Could you check a few things on this model? Use its own coordinates, in mm. Coordinates: 2 decimals unless noted, no trailing zeros. Loops run counter-clockwise (first coordinate to the right, second up) from the corner with the lowest first, then second, coordinate; pieces in that order, holes last. Notation, with made-up numbers: (48.25, 57.5) - (60.25, 57.5) arc R14 ccw to (60.25, 77.5) - close; hole circle Ø8 at (70.25, 32.5). An arc over 180 degrees is marked (long way). One line per item, written item: value. Start each with the question number.
(1) If we section it at A-A on z = 1.6: Count the separate pieces of the cut face and the enclosed holes in it, then the cut area to 3 significant figures.
(2) I'm going to push a flat-ended pin straight in: P1, Ø5.5, axis at x = 320.675, y = 0, coming from the +Z side. Where does the tip first touch, or does it pass through?
(3) If we mould it in two halves opening along X, with no side actions, what happens to faces 1 (the face through (58.89, 6.35, 1.57)), 2 (the face through (308.071, -14.845, 1.565)), 3 (the face through (119, -24, 3.175)), 4 (the face through (-81.46, -97.464, 1.565))? For each: pulls with the +X half, pulls with the -X half, needs draft (parallel to the pull), parting line crosses it, or undercut.
(4) If we section it at B-B on x = 210: Write out the boundary of the cut face in (y, z) (3 decimals).
(5) If I drill on line 1 along Y through (x, z) = (302.5, 2.7); line 2 along X through (y, z) = (0.5, 2.65); line 3 along X through (y, z) = (11, 1.15), over which ranges is the centre line in solid material (lowest first)? Write a range as from..to.
(6) If we section it at C-C on x = -39: Write out the boundary of the cut face in (y, z) (3 decimals).
```python
from build123d import *

# Parameters (mm, degrees)
SKETCH1_R           = 7.9375
SKETCH1_R_2         = 3.429
SKETCH1_R_3         = 14.2875
SKETCH1_R_4         = 3.556
BOSS_EXTRUDE1_DEPTH = 3.175


with BuildPart() as part:
    # Sketch1 → Boss-Extrude1 (new body)
    with BuildSketch(Plane.XY):
        with BuildLine():
            Line((304.8, 25.4), (76.724364717, 25.4))
            ThreePointArc((76.724364717, 25.4), (74.903259532, 24.825807741), (73.740840646, 23.310913955))
            Line((73.740840646, 23.310913955), (70.609033369, 14.70634418))
            ThreePointArc((70.609033369, 14.70634418), (58.674937085, 6.35), (46.740840801, 14.70634418))
            Line((46.740840801, 14.70634418), (43.609033524, 23.310913955))
            ThreePointArc((43.609033524, 23.310913955), (42.446614639, 24.825807741), (40.625509453, 25.4))
            Line((40.625509453, 25.4), (9.593010709, 25.4))
            ThreePointArc((9.593010709, 25.4), (5.643057573, 24.542381105), (2.404401957, 22.123962251))
            Line((2.404401957, 22.123962251), (-83.157756356, -76.304041526))
            ThreePointArc((-83.157756356, -76.304041526), (-83.615224536, -76.995200552), (-83.878219746, -77.781210383))
            Line((-83.878219746, -77.781210383), (-86.451909051, -91.021694031))
            ThreePointArc((-86.451909051, -91.021694031), (-86.337264221, -92.661191482), (-85.418230161, -94.023715509))
            Line((-85.418230161, -94.023715509), (-77.389837916, -101.002690413))
            ThreePointArc((-77.389837916, -101.002690413), (-73.552808487, -103.028646494), (-69.21525712, -103.142405102))
            Line((-69.21525712, -103.142405102), (309.934982787, -24.875529176))
            ThreePointArc((309.934982787, -24.875529176), (330.068542113, 2.580848594), (304.8, 25.4))
        make_face()
        with Locations((304.8, 0)):
            Circle(SKETCH1_R, mode=Mode.SUBTRACT)
        Circle(SKETCH1_R, mode=Mode.SUBTRACT)
        with Locations((-66.655597345, -76.678493351)):
            Circle(SKETCH1_R, mode=Mode.SUBTRACT)
        with Locations((304.8, 15.875)):
            Circle(SKETCH1_R_2, mode=Mode.SUBTRACT)
        with Locations((320.675, 0)):
            Circle(SKETCH1_R_2, mode=Mode.SUBTRACT)
        with Locations((304.8, -15.875)):
            Circle(SKETCH1_R_2, mode=Mode.SUBTRACT)
        with Locations((288.925, 0)):
            Circle(SKETCH1_R_2, mode=Mode.SUBTRACT)
        with Locations((-56.24066026, -64.697478765)):
            Circle(SKETCH1_R_2, mode=Mode.SUBTRACT)
        with Locations((-54.674582759, -87.093430436)):
            Circle(SKETCH1_R_2, mode=Mode.SUBTRACT)
        with Locations((-77.070534431, -88.659507937)):
            Circle(SKETCH1_R_2, mode=Mode.SUBTRACT)
        with Locations((-10.414937085, -11.981014586)):
            Circle(SKETCH1_R_2, mode=Mode.SUBTRACT)
        with Locations((11.981014586, -10.414937085)):
            Circle(SKETCH1_R_2, mode=Mode.SUBTRACT)
        with Locations((10.414937085, 11.981014586)):
            Circle(SKETCH1_R_2, mode=Mode.SUBTRACT)
        with Locations((130.671295769, -35.944879509)):
            Circle(SKETCH1_R_3, mode=Mode.SUBTRACT)
        with Locations((115.786625943, -1.087398892)):
            Circle(SKETCH1_R_4, mode=Mode.SUBTRACT)
    extrude(amount=BOSS_EXTRUDE1_DEPTH)


solid = part.part
```
Values:
1. separate pieces: 1
1. enclosed holes: 15
1. area: 29,900 mm2
2. P1: passes through
3. face 1: undercut
3. face 2: undercut
3. face 3: needs draft
3. face 4: pulls with the -X half
4. outline: (-45.505, 0) - (25.4, 0) - (25.4, 3.175) - (-45.505, 3.175) - close
5. line 1: y = -26.41..-18.42, -13.33..-7.6, 7.6..13.33, 18.42..25.4
5. line 2: x = -16.39..-7.92, 7.92..112.6, 118.97..285.53, 292.32..296.88, 312.72..317.28, 324.07..330.2
5. line 3: x = -7.27..7.13, 13.7..48.85, 68.5..327.69
6. outline: (-96.905, 0) - (-25.506, 0) - (-25.506, 3.175) - (-96.905, 3.175) - close
